from build123d import *

# Parameters (mm, degrees)
SKETCH1_W                  = 106
SKETCH1_H                  = 57
BOSS_EXTRUDE1_DEPTH        = 1.5
CUT_EXTRUDE1_DEPTH         = 61.195514783
CUT_EXTRUDE1_DEPTH_BACK    = 61.195514783
SKETCH2_W                  = 3
SKETCH2_H                  = 22.5
SKETCH2_W_2                = 40
SKETCH2_H_2                = 3
SKETCH4_W                  = 15
SKETCH4_H                  = 9
BOSS_EXTRUDE2_DEPTH        = 1.5
FILLET1_R                  = 2
CUT_EXTRUDE2_DEPTH         = 65.942282066
CUT_EXTRUDE2_DEPTH_BACK    = 65.942282066
CUT_EXTRUDE3_DEPTH         = 65.942282066
CUT_EXTRUDE3_DEPTH_BACK    = 65.942282066
SKETCH5_R                  = 1.5
FILLET2_R                  = 5
CUT_EXTRUDE4_DEPTH         = 65.942282066
CUT_EXTRUDE4_DEPTH_BACK    = 65.942282066
SKETCH6_R                  = 1.5
CORTE_EXTRUS_O1_DEPTH      = 65.994230513
CORTE_EXTRUS_O1_DEPTH_BACK = 65.994230513


with BuildPart() as part:
    # Sketch1 → Boss-Extrude1 (new, symmetric)
    with BuildSketch(Plane(origin=(0, 0, 0), x_dir=(1, 0, 0), z_dir=(0, 1, 0))):
        Rectangle(SKETCH1_W, SKETCH1_H)
    extrude(amount=BOSS_EXTRUDE1_DEPTH, both=True)

    # Sketch2 → Cut-Extrude1 (cut, two sides: drawn at the far end of the back side and taken through both)
    with BuildSketch(Plane(origin=(0, 0, 0), x_dir=(1, 0, 0), z_dir=(0, 1, 0)).offset(-CUT_EXTRUDE1_DEPTH_BACK)):
        with Locations((-51.5, 17.25)):
            Rectangle(SKETCH2_W, SKETCH2_H)
        with Locations((51.5, 17.25)):
            Rectangle(SKETCH2_W, SKETCH2_H)
        with Locations((0, -27)):
            Rectangle(SKETCH2_W_2, SKETCH2_H_2)
    extrude(amount=CUT_EXTRUDE1_DEPTH + CUT_EXTRUDE1_DEPTH_BACK, mode=Mode.SUBTRACT)

    # Sketch4 → Boss-Extrude2 (add, symmetric)
    with BuildSketch(Plane(origin=(0, 0, 0), x_dir=(1, 0, 0), z_dir=(0, 1, 0))):
        with Locations((0, 33)):
            Rectangle(SKETCH4_W, SKETCH4_H)
    extrude(amount=BOSS_EXTRUDE2_DEPTH, both=True)

    # Fillet1
    fillet1_edges = [part.edges().sort_by_distance(p)[0] for p in [
        (-7.5, 0, -37.5),
        (-7.5, 0, -28.5),
        (7.5, 0, -28.5),
        (7.5, 0, -37.5),
    ]]
    fillet(fillet1_edges, radius=FILLET1_R)

    # Sketch3 → Cut-Extrude2 (cut, two sides: drawn at the far end of the back side and taken through both)
    with BuildSketch(Plane(origin=(0, 0, 0), x_dir=(1, 0, 0), z_dir=(0, 1, 0)).offset(-CUT_EXTRUDE2_DEPTH_BACK)):
        with BuildLine():
            Line((-1.5, -25.5), (1.5, -25.5))
            Line((1.5, -25.5), (1.5, -21.5))
            Line((1.5, -21.5), (2.8, -21.5))
            Line((2.8, -21.5), (2.8, -19.23))
            Line((2.8, -19.23), (1.5, -19.23))
            Line((1.5, -19.23), (1.5, -14.5))
            ThreePointArc((1.5, -14.5), (1.207106781, -13.792893219), (0.5, -13.5))
            Line((0.5, -13.5), (-0.5, -13.5))
            ThreePointArc((-0.5, -13.5), (-1.207106781, -13.792893219), (-1.5, -14.5))
            Line((-1.5, -14.5), (-1.5, -19.23))
            Line((-1.5, -19.23), (-2.8, -19.23))
            Line((-2.8, -19.23), (-2.8, -21.5))
            Line((-2.8, -21.5), (-1.5, -21.5))
            Line((-1.5, -21.5), (-1.5, -25.5))
        make_face()
    extrude(amount=CUT_EXTRUDE2_DEPTH + CUT_EXTRUDE2_DEPTH_BACK, mode=Mode.SUBTRACT)

    # Sketch5 → Cut-Extrude3 (cut, two sides: drawn at the far end of the back side and taken through both)
    with BuildSketch(Plane(origin=(0, 0, 0), x_dir=(1, 0, 0), z_dir=(0, 1, 0)).offset(-CUT_EXTRUDE3_DEPTH_BACK)):
        with Locations(Location((0, 33, 0), (0, 0, 270))):
            Circle(SKETCH5_R)
    extrude(amount=CUT_EXTRUDE3_DEPTH + CUT_EXTRUDE3_DEPTH_BACK, mode=Mode.SUBTRACT)

    # Fillet2
    fillet2_edges = [part.edges().sort_by_distance(p)[0] for p in [
        (53, 0, 28.5),
        (-53, 0, 28.5),
    ]]
    fillet(fillet2_edges, radius=FILLET2_R)

    # Sketch6 → Cut-Extrude4 (cut, two sides: drawn at the far end of the back side and taken through both)
    with BuildSketch(Plane(origin=(0, 0, 0), x_dir=(1, 0, 0), z_dir=(0, 1, 0)).offset(-CUT_EXTRUDE4_DEPTH_BACK)):
        with Locations(Location((-4.3, -3, 0), (0, 0, 270))):
            Circle(SKETCH6_R)
        with Locations(Location((4.3, -3, 0), (0, 0, 270))):
            Circle(SKETCH6_R)
        with Locations(Location((10.2, -10.15, 0), (0, 0, 270))):
            Circle(SKETCH6_R)
        with Locations(Location((10.2, -16.25, 0), (0, 0, 270))):
            Circle(SKETCH6_R)
        with Locations(Location((-10.2, -16.25, 0), (0, 0, 90))):
            Circle(SKETCH6_R)
        with Locations(Location((-10.2, -10.15, 0), (0, 0, 90))):
            Circle(SKETCH6_R)
    extrude(amount=CUT_EXTRUDE4_DEPTH + CUT_EXTRUDE4_DEPTH_BACK, mode=Mode.SUBTRACT)

    # Esboço1 → Corte-extrusão1 (cut, two sides: drawn at the far end of the back side and taken through both)
    with BuildSketch(Plane(origin=(0, 1.5, 0), x_dir=(1, 0, 0), z_dir=(0, 1, 0)).offset(-CORTE_EXTRUS_O1_DEPTH_BACK)):
        with BuildLine():
            Line((-20, -3.9), (-17, -3.9))
            ThreePointArc((-17, -3.9), (-16.292893219, -4.192893219), (-16, -4.9))
            Line((-16, -4.9), (-16, -21.5))
            ThreePointArc((-16, -21.5), (-16.292893219, -22.207106781), (-17, -22.5))
            Line((-17, -22.5), (-20, -22.5))
            ThreePointArc((-20, -22.5), (-20.707106781, -22.207106781), (-21, -21.5))
            Line((-21, -21.5), (-21, -4.9))
            ThreePointArc((-21, -4.9), (-20.707106781, -4.192893219), (-20, -3.9))
        make_face()
        with BuildLine():
            Line((21, -4.9), (21, -21.5))
            ThreePointArc((21, -21.5), (20.707106781, -22.207106781), (20, -22.5))
            Line((20, -22.5), (17, -22.5))
            ThreePointArc((17, -22.5), (16.292893219, -22.207106781), (16, -21.5))
            Line((16, -21.5), (16, -4.9))
            ThreePointArc((16, -4.9), (16.292893219, -4.192893219), (17, -3.9))
            Line((17, -3.9), (20, -3.9))
            ThreePointArc((20, -3.9), (20.707106781, -4.192893219), (21, -4.9))
        make_face()
    extrude(amount=CORTE_EXTRUS_O1_DEPTH + CORTE_EXTRUS_O1_DEPTH_BACK, mode=Mode.SUBTRACT)


solid = part.part
Check sheet for the modelled part. Datum: model origin and axes. Units: mm. A direction names the side the tool comes from. Give positions to 0.01 mm unless a question says otherwise; leave off trailing zeros. Order: outer loops, then holes, each group sorted by start corner. A loop starts at its lowest first (then second) coordinate and runs counter-clockwise, first axis right, second up. Notation, with made-up numbers: (29, 83.5) - (77, 83.5) arc R10 ccw to (77, 88.5) - close; hole circle Ø7 at (26.25, 89). An arc over 180 degrees is marked (long way). Answer as CSV lines item,"result".
1. Section check C-C (y = 0.5). State how many separate pieces and enclosed holes the cut face has, then the cut area to 3 significant figures.
Result sheet:
separate pieces,"1"
enclosed holes,"9"
area,"5,640 mm²"
2. Scan lines: probe 1 along Z at (x, y) = (10.2, -0.4); probe 2 along X at (y, z) = (0.4, 3); probe 3 along X at (y, z) = (-0.25, 16.25). Record each from-to range of solid material in increasing order. Write a range as from..to.
Result sheet:
probe 1,"-28.5..8.65, 11.65..14.75, 17.75..25.5"
probe 2,"-53..-5.8, -2.8..2.8, 5.8..53"
probe 3,"-53..-21, -16..-11.7, -8.7..-1.5, 1.5..8.7, 11.7..16, 21..53"
3. Go/stop test with flat-tipped pins: P1, Ø0.9, axis at x = -18, y = 0, coming from the -Z side; P2, Ø1.5, axis at y = 0, z = -17, coming from the -X side; P3, Ø0.9, axis at x = 9, y = 0.5, coming from the +Z side. Record where each tip stops, or that it passes through.
Result sheet:
P1,"z = -28.5"
P2,"x = -50"
P3,"z = 25.5"
4. Tool access check on faces 5 (the face through (-1.5, 0, 17)), 6 (the face through (-21, 0, 13)), 7 (the face through (0, 0, -37.5)), 8 (the face through (7.5, 0, -33)), 9 (the face through (-7.5, 0, -33)). Record the directions out of +Z, -Z, +X, -X, +Y, -Y that give a thin tool (end or side, any length) a straight path to the whole face; none if there is none.
Result sheet:
face 5,"+Z, +Y, -Y"
face 6,"+Y, -Y"
face 7,"-Z, +X, -X, +Y, -Y"
face 8,"-Z, +X, +Y, -Y"
face 9,"-Z, -X, +Y, -Y"
5. Section check A-A (x = 4.3). Record the boundary of the cut face in (y, z), then the cut area to 3 significant figures.
Result sheet:
outline,"(-1.5, -37.5) - (1.5, -37.5) - (1.5, 1.5) - (-1.5, 1.5) - close; (-1.5, 4.5) - (1.5, 4.5) - (1.5, 25.5) - (-1.5, 25.5) - close"
area,"180 mm²"
6. Section check B-B (z = 10). Record the boundary of the cut face in (x, y).
Result sheet:
outline,"(-53, -1.5) - (-21, -1.5) - (-21, 1.5) - (-53, 1.5) - close; (-16, -1.5) - (-11.69, -1.5) - (-11.69, 1.5) - (-16, 1.5) - close; (-8.71, -1.5) - (8.71, -1.5) - (8.71, 1.5) - (-8.71, 1.5) - close; (11.69, -1.5) - (16, -1.5) - (16, 1.5) - (11.69, 1.5) - close; (21, -1.5) - (53, -1.5) - (53, 1.5) - (21, 1.5) - close"
7. Mould release check, pull along X, two halves, no side actions. Record for faces 1 (the face through (51, 0, -6)), 2 (the face through (21, 0, 13)), 3 (the face through (16, 0, 13)), 4 (the face through (51.57, 0.02, 27)): released by +X, released by -X, zero draft, split by the parting line, or undercut.
Result sheet:
face 1,"zero draft"
face 2,"undercut"
face 3,"undercut"
face 4,"released by +X"
8. Section check D-D (z = 2.5). Record the boundary of the cut face in (x, y), then the cut area to 3 significant figures.
Result sheet:
outline,"(-53, -1.5) - (-5.71, -1.5) - (-5.71, 1.5) - (-53, 1.5) - close; (-2.89, -1.5) - (2.89, -1.5) - (2.89, 1.5) - (-2.89, 1.5) - close; (5.71, -1.5) - (53, -1.5) - (53, 1.5) - (5.71, 1.5) - close"
area,"301 mm²"
